Can you work these out from the model? Positions are in its coordinate system, mm. A direction names the side the tool comes from. Round coordinates to 2 decimals unless told otherwise and drop trailing zeros. Loops run counter-clockwise (first coordinate to the right, second up) from the corner with the lowest first, then second, coordinate; pieces in that order, holes last.
(1) Thinking about a two-plate mould opening in Z: for faces 1 (the face through (1, 9.5, 9)), 2 (the face through (4.07, 1.01, -6.2)), 3 (the face through (1.6, 4.4, -13.5)), which applies, released by +Z, released by -Z, zero draft, split by the parting line, or undercut?
(2) I want a section at C-C on y = 9.25. Write out the boundary of the cut face in (x, z), plus the area to 3 significant figures.
(3) Will these pins go through, and if not, where does the flat tip stop? pin 1 Ø1.8 at (x, z) = (4, -4.7) entering from +Y; pin 2 Ø0.8 at (x, y) = (1.5, 10.5) entering from +Z; pin 3 Ø3 at (x, y) = (4, 6.5) entering from +Z; pin 4 Ø2 at (x, z) = (1, 6.5) entering from +Y.
(4) I want a section at D-D on x = 4. Write out the boundary of the cut face in (y, z), plus the area to 3 significant figures.
(5) Which directions (+Z, -Z, +X, -X, +Y, -Y) give clear straight access to the entire face, cutting with the end or side of a thin tool? Please do faces 4 (the face through (3, 4, -2)), 5 (the face through (3, 4, 0)), 6 (the face through (1, 10, 3.5)), 7 (the face through (4, 1, 9.5)).
(6) I want a section at B-B on z = -4.7. Write out the boundary of the cut face in (x, y), plus the area to 3 significant figures.
(7) I want a section at A-A on y = 1.75. Write out the boundary of the cut face in (x, z).
(8) If I drill on line 1 along Z through (x, y) = (1.15, 9.25); line 2 along Z through (x, y) = (4.85, 1.75); line 3 along Y through (x, z) = (1.9, 11.75), over which ranges is the centre line in solid material (lowest first)?
from build123d import *

# Parameters (mm, degrees)
BOSS_EXTRUDE1_DEPTH = 13.5
SKETCH2_W           = 10
SKETCH2_H           = 1.5
CUT_EXTRUDE1_DEPTH  = 27
SKETCH3_R           = 1
CUT_EXTRUDE2_DEPTH  = 3.6
SKETCH6_W           = 6
SKETCH6_H           = 2
BOSS_EXTRUDE2_DEPTH = 3
SKETCH7_R           = 1.5
CUT_EXTRUDE5_DEPTH  = 9
BOSS_EXTRUDE3_DEPTH = 2
SKETCH10_W          = 6
SKETCH10_H          = 3
CUT_EXTRUDE6_DEPTH  = 10
SKETCH11_W          = 4
SKETCH11_H          = 4
CUT_EXTRUDE7_DEPTH  = 10


with BuildPart() as part:
    # Sketch1 → Boss-Extrude1 (new, symmetric)
    with BuildSketch(Plane.XY):
        Polygon((0, 11), (0, 0), (6, 0), (6, 2), (2, 2), (2, 11), align=None)
    extrude(amount=BOSS_EXTRUDE1_DEPTH, both=True)

    # Sketch2 → Cut-Extrude1 (cut)
    with BuildSketch(Plane(origin=(2, 0, 0), x_dir=(0, 0, -1), z_dir=(1, 0, 0))):
        with Locations((-8.5, 10.25)):
            Rectangle(SKETCH2_W, SKETCH2_H)
    extrude(amount=-CUT_EXTRUDE1_DEPTH, mode=Mode.SUBTRACT)

    # Sketch3 → Cut-Extrude2 (cut)
    with BuildSketch(Plane.ZY):
        with Locations(Location((-11.75, 9.25, 0), (0, 0, 270))):
            Circle(SKETCH3_R)
        with Locations(Location((11.723777669, 1.75, 0), (0, 0, 270))):
            Circle(SKETCH3_R)
    extrude(amount=-CUT_EXTRUDE2_DEPTH, mode=Mode.SUBTRACT)

    # Sketch6 → Boss-Extrude2 (add)
    with BuildSketch(Plane(origin=(0, 0, -13.5), x_dir=(-1, 0, 0), z_dir=(0, 0, -1))):
        with Locations((-3, 1)):
            Rectangle(SKETCH6_W, SKETCH6_H)
    extrude(amount=BOSS_EXTRUDE2_DEPTH)

    # Sketch7 → Cut-Extrude5 (cut)
    with BuildSketch(Plane(origin=(0, 2, 0), x_dir=(1, 0, 0), z_dir=(0, 1, 0))):
        with Locations(Location((4, -4.7, 0), (0, 0, 180))):
            Circle(SKETCH7_R)
        with Locations(Location((4, 4.7, 0), (0, 0, 270))):
            Circle(SKETCH7_R)
    extrude(amount=-CUT_EXTRUDE5_DEPTH, mode=Mode.SUBTRACT)

    # Sketch9 → Boss-Extrude3 (add)
    with BuildSketch(Plane.XY):
        Polygon((2, 8.5), (2, 2), (6, 2), align=None)
    extrude(amount=-BOSS_EXTRUDE3_DEPTH)

    # Sketch10 → Cut-Extrude6 (cut)
    with BuildSketch(Plane(origin=(0, 2, 0), x_dir=(1, 0, 0), z_dir=(0, 1, 0))):
        with Locations((3, 15)):
            Rectangle(SKETCH10_W, SKETCH10_H)
    extrude(amount=-CUT_EXTRUDE6_DEPTH, mode=Mode.SUBTRACT)

    # Sketch11 → Cut-Extrude7 (cut)
    with BuildSketch(Plane(origin=(0, 2, 0), x_dir=(1, 0, 0), z_dir=(0, 1, 0))):
        with Locations((4, -11.5)):
            Rectangle(SKETCH11_W, SKETCH11_H)
    extrude(amount=-CUT_EXTRUDE7_DEPTH, mode=Mode.SUBTRACT)


solid = part.part
Filled sheet:
1. face 1: zero draft
1. face 2: undercut
1. face 3: released by -Z
2. outline: (0, -13.5) - (2, -13.5) - (2, -12.75) - (0, -12.75) - close; (0, -10.75) - (2, -10.75) - (2, 13.5) - (0, 13.5) - close
2. area: 50.0 mm2
3. pin 1: passes through
3. pin 2: stops at z = 3.5
3. pin 3: stops at z = 0
3. pin 4: stops at y = 9.5
4. outline: (0, -13.5) - (2, -13.5) - (2, -6.2) - (0, -6.2) - close; (0, -3.2) - (2, -3.2) - (2, -2) - (5.25, -2) - (5.25, 0) - (2, 0) - (2, 3.2) - (0, 3.2) - close; (0, 6.2) - (2, 6.2) - (2, 9.5) - (0, 9.5) - close
4. area: 40.5 mm2
5. face 4: -Z, +X, +Y
5. face 5: +Z, +X, +Y
5. face 6: +Z, +X, -X, +Y
5. face 7: +Z, +X, +Y, -Y
6. outline: (0, 0) - (2.5, 0) - (2.5, 2) - (2, 2) - (2, 11) - (0, 11) - close; (5.5, 0) - (6, 0) - (6, 2) - (5.5, 2) - close
6. area: 24.0 mm2
7. outline: (0, -13.5) - (6, -13.5) - (6, 9.5) - (2, 9.5) - (2, 10.72) - (0, 10.72) - close; (0, 12.72) - (2, 12.72) - (2, 13.5) - (0, 13.5) - close; hole circle Ø3 at (4, -4.7); hole circle Ø3 at (4, 4.7)
8. line 1: z = -13.5 to -12.75, -10.75 to 13.5
8. line 2: z = -13.5 to -5.94, -3.46 to 3.46, 5.94 to 9.5
8. line 3: y = 0 to 0.75, 2.75 to 9.5
